Design review of the part built by this model. Coordinates are the model's own, in mm. A direction names the side the tool comes from. Coordinates: 2 decimals unless noted, no trailing zeros. Write each loop counter-clockwise with the first axis right and the second up, starting at its lowest first coordinate (ties: lowest second). Pieces come first, ordered by that corner, then holes.
Q1. Take a section at C-C (x = 0). Give the boundary of the cut face in (y, z).
Q2. Insertion check: pin 1 (2.5 mm diameter, centred on x = -2, z = 0.5, fed in from -Y); pin 2 (3 mm diameter, centred on x = 1, z = -1, fed in from -Y). Each pin has a flat end and moves straight along its axis. Give the tip position at first contact, or say it passes through.
Q3. Mouldability with a two-part tool opening along Z and no side actions: class faces 3 (the cylindrical face through (-0.026, 7.768, -9.238)), 4 (the flat face through (0, 16, 0)), 5 (the cylindrical face through (1.352, 2.071, -4.292)) as pulls with the +Z half, pulls with the -Z half, needs draft (parallel to the pull), parting line crosses it, or undercut.
Q4. For probe 1 along X at (y, z) = (3, 0); probe 2 along X at (y, z) = (12.5, 0); probe 3 along X at (y, z) = (12, -4.5), list the stretches that pass through material, from the lowest coordinate up.
Q5. Machinability: for faces 1 (the cylindrical face through (-0.06, 7.42, 9.75)), 2 (the cylindrical face through (0.9, 9.52, -2.86)), which of the approach directions +Z, -Z, +X, -X, +Y, -Y give a long, thin tool a straight path to every point of the face, cutting with its end or side? Answer none if there is none.
Q6. Take a section at A-A (z = 0). Give the boundary of the cut face in (x, y), and give its area (3 significant figures).
```python
from build123d import *

# Parameters (mm, degrees)
SKETCH1_R           = 9.75
BOSS_EXTRUDE1_DEPTH = 16
SKETCH2_R           = 3
CUT_EXTRUDE1_DEPTH  = 15
SKETCH5_R           = 4.5
CUT_EXTRUDE2_DEPTH  = 4.2
FILLET1_R           = 3
FILLET2_R           = 2
SKETCH11_R          = 4.7625
CUT_EXTRUDE4_DEPTH  = 17
CIRPATTERN3_COUNT   = 5


with BuildPart() as part:
    # Sketch1 → Boss-Extrude1 (new body)
    with BuildSketch(Plane(origin=(0, 0, 0), x_dir=(1, 0, 0), z_dir=(0, 1, 0))):
        with Locations(Location((0, 0, 0), (0, 0, 90))):  # turned: the seam where the file's is
            Circle(SKETCH1_R)
    extrude(amount=BOSS_EXTRUDE1_DEPTH)

    # Sketch2 → Cut-Extrude1 (cut)
    with BuildSketch(Plane.XZ):
        with Locations(Location((0, 0, 0), (0, 0, 270))):  # turned: the seam where the file's is
            Circle(SKETCH2_R)
    extrude(amount=-CUT_EXTRUDE1_DEPTH, mode=Mode.SUBTRACT)

    # Sketch5 → Cut-Extrude2 (cut)
    with BuildSketch(Plane.XZ):
        with Locations(Location((0, 0, 0), (0, 0, 270))):  # turned: the seam where the file's is
            Circle(SKETCH5_R)
    extrude(amount=-CUT_EXTRUDE2_DEPTH, mode=Mode.SUBTRACT)

    # Fillet1
    fillet1_edges = [part.edges().sort_by_distance(p)[0] for p in [
        (0, 16, 9.75),
    ]]
    fillet(fillet1_edges, radius=FILLET1_R)

    # Fillet2
    fillet2_edges = [part.edges().sort_by_distance(p)[0] for p in [
        (0, 0, 9.75),
    ]]
    fillet(fillet2_edges, radius=FILLET2_R)

    # Sketch11 → Cut-Extrude4 (cut, through all)
    with BuildSketch(Plane(origin=(0, 16, 0), x_dir=(1, 0, 0), z_dir=(0, 1, 0))):
        with Locations((0, 14)):
            Circle(SKETCH11_R)
    cut_extrude4 = extrude(amount=-CUT_EXTRUDE4_DEPTH, mode=Mode.SUBTRACT)

    # CirPattern3: Cut-Extrude4 ×5 about axis
    cirpattern3_axis = Axis((0, 0, 0), (0, 1, 0))
    for i in range(1, CIRPATTERN3_COUNT):
        add(cut_extrude4.rotate(cirpattern3_axis, i * 360 / CIRPATTERN3_COUNT), mode=Mode.SUBTRACT)


solid = part.part
```
Response:
1. outline: (0, -7.75) arc R2 ccw to (0.66, -9.24) - (14.68, -9.24) arc R3 ccw to (16, -6.75) - (16, 6.75) arc R3 ccw to (13, 9.75) - (2, 9.75) arc R2 ccw to (0, 7.75) - (0, 4.5) - (4.2, 4.5) - (4.2, 3) - (15, 3) - (15, -3) - (4.2, -3) - (4.2, -4.5) - (0, -4.5) - close
2. pin 1: stops at y = 4.2
2. pin 2: stops at y = 15
3. face 3: pulls with the -Z half
3. face 4: needs draft
3. face 5: undercut
4. probe 1: x = -9.75 to -4.5, 4.5 to 9.75
4. probe 2: x = -9.75 to -3, 3 to 9.75
4. probe 3: x = -8.56 to 8.56
5. face 1: +Z, +Y, -Y
5. face 2: -Y
6. outline: (-9.75, 2) arc R2 ccw to (-7.75, 0) - (-4.5, 0) - (-4.5, 4.2) - (-3, 4.2) - (-3, 15) - (3, 15) - (3, 4.2) - (4.5, 4.2) - (4.5, 0) - (7.75, 0) arc R2 ccw to (9.75, 2) - (9.75, 13) arc R3 ccw to (6.75, 16) - (-6.75, 16) arc R3 ccw to (-9.75, 13) - close
6. area: 204 mm2
